```python
from build123d import *

# Parameters (mm, degrees)
BOSS_EXTRUDE1_DEPTH             = 7.5
BOSS_EXTRUDE1_DEPTH_BACK        = 7.5
SKETCH2_W                       = 25
SKETCH2_H                       = 52.5
BOSS_EXTRUDE2_DEPTH             = 2
F_3_0MM_DOWEL_HOLE1_D           = 3
F_3_0MM_DOWEL_HOLE1_CSINK_D     = 3.05
F_3_0MM_DOWEL_HOLE1_CSINK_ANGLE = 90


with BuildPart() as part:
    # Sketch1 → Boss-Extrude1 (new, two sides: drawn at the far end of the back side and taken through both)
    with BuildSketch(Plane.YZ.offset(-BOSS_EXTRUDE1_DEPTH_BACK)):
        Polygon((-10.75, -21.25), (-10.75, 21.25), (-12.5, 21.25), (-12.5, -31.25), (12.5, -31.25), (12.5, 21.25), (10.75, 21.25), (10.75, -15.25), (-2.25, -15.25), (-2.25, -21.25), align=None)
    extrude(amount=BOSS_EXTRUDE1_DEPTH + BOSS_EXTRUDE1_DEPTH_BACK)

    # Sketch2 → Boss-Extrude2 (add)
    with BuildSketch(Plane.YZ.offset(7.5)):
        with Locations((0, -5)):
            Rectangle(SKETCH2_W, SKETCH2_H)
    boss_extrude2 = extrude(amount=BOSS_EXTRUDE2_DEPTH)

    # Mirror2: Boss-Extrude2 across plane
    add(boss_extrude2.mirror(Plane(origin=(0, 0, 0), x_dir=(0, 0, 1), z_dir=(1, 0, 0))))

    # Ø3.0mm Dowel Hole1 (through all)
    with Locations(Plane.YZ.offset(9.5)):
        with Locations((2.25, 20.85), (-5.25, -18.25)):
            CounterSinkHole(F_3_0MM_DOWEL_HOLE1_D / 2, F_3_0MM_DOWEL_HOLE1_CSINK_D / 2, counter_sink_angle=F_3_0MM_DOWEL_HOLE1_CSINK_ANGLE)


solid = part.part
```
Part model, mm, in its own coordinate system. A direction names the side the tool comes from. Round coordinates to 2 decimals unless told otherwise and drop trailing zeros. Write each loop counter-clockwise with the first axis right and the second up, starting at its lowest first coordinate (ties: lowest second). Pieces come first, ordered by that corner, then holes.
Item 1: Drop flat-ended pins along their axis: pin 1 Ø4 at (x, y) = (3, -5) entering from +Z; pin 2 Ø6.5 at (x, y) = (-0.5, 4) entering from +Z; pin 3 Ø2.5 at (y, z) = (2.25, 20.85) entering from -X. Give the stop position or say it passes through.
Results:
pin 1: stops at z = -21.25
pin 2: stops at z = -15.25
pin 3: passes through
Item 2: Two-plate mould, pull along X, no slides. Class faces 1 (the flat face through (0, 11, 21.25)), 2 (the flat face through (9.5, 0, -5)), 3 (the flat face through (7.5, 0, 0)): +X half, -X half, draft (parallel to the pull), parting line (faces both ways), or undercut.
Results:
face 1: draft
face 2: +X half
face 3: undercut
Item 3: Cut at C-C, the plane x = -1.25. Give the cut face in (y, z).
Results:
outline: (-12.5, -31.25) - (12.5, -31.25) - (12.5, 21.25) - (10.75, 21.25) - (10.75, -15.25) - (-2.25, -15.25) - (-2.25, -21.25) - (-10.75, -21.25) - (-10.75, 21.25) - (-12.5, 21.25) - close
Item 4: Probe L1, parallel to Z at x = -8.45, y = -5.25; L2, parallel to X at y = 1.5, z = -10; L3, parallel to Y at x = -0.5, z = -13. List the from-to ranges inside material, lowest first.
Results:
L1: z = -31.25 to -19.75, -16.75 to 21.25
L2: x = -9.5 to -7.5, 7.5 to 9.5
L3: y = -12.5 to -10.75, 10.75 to 12.5
Item 5: Cut at D-D, the plane z = -11. Give the cut face in (x, y).
Results:
outline: (-9.5, -12.5) - (9.5, -12.5) - (9.5, 12.5) - (-9.5, 12.5) - close; hole (-7.5, -10.75) - (7.5, -10.75) - (7.5, 10.75) - (-7.5, 10.75) - close
Item 6: Cut at B-B, the plane y = -5.25. Give the cut face in (x, z) (3 decimals), plus the area to 3 significant figures.
Results:
outline: (-9.5, -31.25) - (9.5, -31.25) - (9.5, -19.775) - (9.475, -19.75) - (7.5, -19.75) - (7.5, -21.25) - (-7.5, -21.25) - (-7.5, -19.75) - (-9.5, -19.75) - close; (-9.5, -16.75) - (-7.5, -16.75) - (-7.5, 21.25) - (-9.5, 21.25) - close; (7.5, -16.75) - (9.475, -16.75) - (9.5, -16.725) - (9.5, 21.25) - (7.5, 21.25) - close
area: 348 mm2
Item 7: Which spindle directions (+Z, -Z, +X, -X, +Y, -Y) get a long thin tool onto all of the face, cutting with end or side? Do faces 4 (the cylindrical face through (8.47, 2.29, 19.35)), 5 (the flat face through (0, 10.75, 3)). Say none if no direction does.
Results:
face 4: +X, -X
face 5: +Z
Item 8: Cut at A-A, the plane z = -18.25. Give the cut face in (x, y) (3 decimals), plus the area to 4 significant figures.
Results:
outline: (-9.5, -12.5) - (9.5, -12.5) - (9.5, -6.775) - (9.475, -6.75) - (7.5, -6.75) - (7.5, -10.75) - (-7.5, -10.75) - (-7.5, -6.75) - (-9.5, -6.75) - close; (-9.5, -3.75) - (-7.5, -3.75) - (-7.5, -2.25) - (7.5, -2.25) - (7.5, -3.75) - (9.475, -3.75) - (9.5, -3.725) - (9.5, 12.5) - (-9.5, 12.5) - close
area: 335.5 mm2
